```python
from build123d import *

# Parameters (mm, degrees)
F0_R      = 1.75
F0_R_2    = 12
F1_DEPTH  = 2.3
F2_DEPTH  = 5.1
F3_W      = 14.9775519967
F3_H      = 15.6408976763
F3_W_2    = 4.8427809961
F3_H_2    = 1.104
F4_DEPTH  = 1
F5_DEPTH  = 3
F6_SIZE   = 1.5
F7_W      = 14.5
F7_H      = 16
F8_DEPTH  = 28
F9_W      = 4.4338763691
F9_H      = 4.8907462656
F10_DEPTH = 8
F11_DEPTH = 30.1


with BuildPart() as f1:
    # F0 (on Front) → F1 (new body)
    with BuildSketch(Plane.XZ):
        with BuildLine():
            ThreePointArc((13, 12), (11.9748737342, 14.4748737342), (9.5, 15.5))
            Line((9.5, 15.5), (-9.5, 15.5))
            ThreePointArc((-9.5, 15.5), (-11.9748737342, 14.4748737342), (-13, 12))
            Line((-13, 12), (-13, -12))
            ThreePointArc((-13, -12), (-11.9748737342, -14.4748737342), (-9.5, -15.5))
            Line((-9.5, -15.5), (9.5, -15.5))
            ThreePointArc((9.5, -15.5), (11.9748737342, -14.4748737342), (13, -12))
            Line((13, -12), (13, 12))
        make_face()
        with Locations((9.5, -12)):
            Circle(F0_R, mode=Mode.SUBTRACT)
        with Locations((-9.5, 12)):
            Circle(F0_R, mode=Mode.SUBTRACT)
        Circle(F0_R_2, mode=Mode.SUBTRACT)
        Circle(F0_R_2)
    extrude(amount=F1_DEPTH)

    # F0 (on Front) → F2 (join)
    with BuildSketch(Plane.XZ):
        Circle(F0_R_2)
    extrude(amount=F2_DEPTH)

    # F3 (on face) → F4 (cut)
    with BuildSketch(Plane.XZ.offset(5.1)):
        Rectangle(F3_W, F3_H)
        Polygon((-4.5, 3.2868520357), (4.5, 3.2868520357), (4.5, -3.2868520357), (2.4213904981, -3.2868520357), (2.4213904981, -4.3908520357), (-2.4213904981, -4.3908520357), (-2.4213904981, -3.2868520357), (-4.5, -3.2868520357), align=None, mode=Mode.SUBTRACT)
        Polygon((4.5, -3.2868520357), (4.5, 3.2868520357), (-4.5, 3.2868520357), (-4.5, -3.2868520357), (-2.4213904981, -3.2868520357), (-2.4213904981, -2.1828520357), (2.4213904981, -2.1828520357), (2.4213904981, -3.2868520357), align=None)
        with Locations((0, -2.7348520357)):
            Rectangle(F3_W_2, F3_H_2)
        with Locations((0, -3.8388520357)):
            Rectangle(F3_W_2, F3_H_2)
    extrude(amount=-F4_DEPTH, mode=Mode.SUBTRACT)

    # F3 (on face) → F5 (cut)
    with BuildSketch(Plane.XZ.offset(5.1)):
        Polygon((4.5, -3.2868520357), (4.5, 3.2868520357), (-4.5, 3.2868520357), (-4.5, -3.2868520357), (-2.4213904981, -3.2868520357), (-2.4213904981, -2.1828520357), (2.4213904981, -2.1828520357), (2.4213904981, -3.2868520357), align=None)
        with Locations((0, -2.7348520357)):
            Rectangle(F3_W_2, F3_H_2)
        with Locations((0, -3.8388520357)):
            Rectangle(F3_W_2, F3_H_2)
    extrude(amount=-F5_DEPTH, mode=Mode.SUBTRACT)

    # F6
    f6_edges = [f1.edges().sort_by_distance(p)[0] for p in [
        (-11.25, -2.3, 12),
        (7.75, -2.3, -12),
    ]]
    chamfer(f6_edges, length=F6_SIZE)

    # F7 (on face) → F8 (join)
    with BuildSketch(Plane(origin=(0, 0, 0), x_dir=(-1, 0, 0), z_dir=(0, 1, 0))):
        Rectangle(F7_W, F7_H)
    extrude(amount=F8_DEPTH)

    # F9 (on face) → F10 (join)
    with BuildSketch(Plane(origin=(0, 0, 0), x_dir=(-1, 0, 0), z_dir=(0, 1, 0))):
        with Locations((0, 8)):
            Rectangle(F9_W, F9_H)
    extrude(amount=F10_DEPTH)

    # F11 (cut, through all): a face of the model
    f11_faces = [f1.faces().sort_by_distance(p)[0] for p in [
        (0, -2.1, -0.3181557698),
    ]]
    extrude(f11_faces, amount=-F11_DEPTH, mode=Mode.SUBTRACT)


solid = f1.part
```
The listing builds one solid part. Answer for the finished solid, in the listing's coordinates (mm). A direction names the side the tool comes from. Give positions to 0.01 mm unless a question says otherwise; leave off trailing zeros. Order: outer loops, then holes, each group sorted by start corner. A loop starts at its lowest first (then second) coordinate and runs counter-clockwise, first axis right, second up. Notation, with made-up numbers: (44.25, -6) -> (51.25, -6) arc R7 ccw to (51.25, 6) -> close; hole circle Ø4 at (63, -3). An arc over 180 degrees is marked (long way). Write each question's results on one line, items separated by ' | '.
Q1. The part is cut by section D-D, the plane z = 4.5. Give the vertices of the cut face in (x, y), and give its area (3 significant figures).
Checked values:
outline: (-13, -2.3) -> (-11.12, -2.3) -> (-11.12, -5.1) -> (-7.49, -5.1) -> (-7.49, -4.1) -> (7.49, -4.1) -> (7.49, -5.1) -> (11.12, -5.1) -> (11.12, -2.3) -> (13, -2.3) -> (13, 0) -> (7.25, 0) -> (7.25, 28) -> (-7.25, 28) -> (-7.25, 0) -> (-13, 0) -> close | area: 513 mm^2
Q2. The part is cut by section B-B, the plane x = 0. Give the vertices of the cut face in (y, z), and give its area (3 significant figures).
Checked values:
outline: (-5.1, -12) -> (-2.3, -12) -> (-2.3, -15.5) -> (0, -15.5) -> (0, -8) -> (28, -8) -> (28, -4.39) -> (-4.1, -4.39) -> (-4.1, -7.82) -> (-5.1, -7.82) -> close; (-5.1, 7.82) -> (-4.1, 7.82) -> (-4.1, 3.29) -> (28, 3.29) -> (28, 8) -> (8, 8) -> (8, 10.45) -> (0, 10.45) -> (0, 15.5) -> (-2.3, 15.5) -> (-2.3, 12) -> (-5.1, 12) -> close | area: 344 mm^2
Q3. The part is cut by section A-A, the plane y = 10.5. Give the vertices of the cut face in (x, z).
Checked values:
outline: (-7.25, -8) -> (7.25, -8) -> (7.25, 8) -> (-7.25, 8) -> close; hole (-4.5, -3.29) -> (-2.42, -3.29) -> (-2.42, -4.39) -> (2.42, -4.39) -> (2.42, -3.29) -> (4.5, -3.29) -> (4.5, 3.29) -> (-4.5, 3.29) -> close
Q4. Straight lines are drawn through the part: probe 1 along X at (y, z) = (18.5, -2.5); probe 2 along Z at (x, y) = (9.5, -0.45); probe 3 along Z at (x, y) = (-3.75, 11). For each, find the intervals that lie inside material, in ascending order. Write a range as from..to.
Checked values:
probe 1: x = -7.25..-4.5, 4.5..7.25 | probe 2: z = -15.5..-13.75, -10.25..15.5 | probe 3: z = -8..-3.29, 3.29..8
Q5. Determine the mould class of faces 1 (the face through (-2.217, 4, 9)), 2 (the face through (0, -4.1, 4)), 3 (the face through (11.95, -1.13, -14.5)) for opening direction X: pulls with the +X half, pulls with the -X half, needs draft (parallel to the pull), parting line crosses it, or undercut.
Checked values:
face 1: pulls with the -X half | face 2: undercut | face 3: pulls with the +X half
Q6. The part is cut by section C-C, the plane x = -4. Give the vertices of the cut face in (y, z).
Checked values:
outline: (-5.1, -11.31) -> (-2.3, -11.31) -> (-2.3, -15.5) -> (0, -15.5) -> (0, -8) -> (28, -8) -> (28, -3.29) -> (-4.1, -3.29) -> (-4.1, -7.82) -> (-5.1, -7.82) -> close; (-5.1, 7.82) -> (-4.1, 7.82) -> (-4.1, 3.29) -> (28, 3.29) -> (28, 8) -> (0, 8) -> (0, 15.5) -> (-2.3, 15.5) -> (-2.3, 11.31) -> (-5.1, 11.31) -> close
Q7. Each of these flat-tipped pins is pushed along its axis until it touches: P1, Ø1.1, axis at y = -5, z = 3, coming from the +X side; P2, Ø4, axis at x = 9.5, z = -12, coming from the +Y side; P3, Ø2, axis at y = 2.5, z = 9.5, coming from the +X side. Where does it stop, or does it pass through?
Checked values:
P1: stops at x = 11.75 | P2: stops at y = 0 | P3: stops at x = 2.22
Q8. Which of the six approach directions +Z, -Z, +X, -X, +Y, -Y give full straight-line access (tool end or side, diameter ignored) to faces 4 (the face through (7.25, 14, 0)), 5 (the face through (-11.99, -3.68, 0.53)), 6 (the face through (0, 8, 9)), 7 (the face through (0, 12, 3.287))?
Checked values:
face 4: +Z, -Z, +X, +Y | face 5: -Y | face 6: +Z, +X, -X, +Y | face 7: +Y, -Y
